from build123d import *

# Parameters (mm, degrees)
F2_SIZE  = 1
F3_R     = 0.99999
F4_R     = 2
F5_R     = 2
F6_DEPTH = 30.0010001


# Not quite as in the source:
# - a fillet or chamfer is up to 0.001 mm smaller than in the source, because OpenCascade refuses the exact size


with BuildPart() as f1:
    # F0 (on Front) → F1 (revolve)
    with BuildSketch(Plane.XZ):
        Polygon((0, 30), (0, 20), (1, 20), (1, 10), (12, 10), (12, 17.5), (6.3493649054, 17.5), (3, 30), align=None)
    revolve(axis=Axis((7.1844396027, 0, 0), (1, 0, 0)))

    # F2
    f2_edges = [f1.edges().sort_by_distance(p)[0] for p in [
        (12, 0, -17.5),
    ]]
    chamfer(f2_edges, length=F2_SIZE)

    # F3 (radius 1 in the source; OpenCascade refuses exactly that, so slightly less here)
    f3_edges = [f1.edges().sort_by_distance(p)[0] for p in [
        (3, 0, -30),
        (1, 0, -20),
    ]]
    fillet(f3_edges, radius=F3_R)

    # F4
    f4_edges = [f1.edges().sort_by_distance(p)[0] for p in [
        (6.349365, 0, -17.5),
    ]]
    fillet(f4_edges, radius=F4_R)

    # F5 (on Top) → F6 (cut, through all)
    with BuildSketch(Plane.XY):
        with Locations((8, 0)):
            Circle(F5_R)
    extrude(amount=F6_DEPTH, mode=Mode.SUBTRACT)


solid = f1.part
Geometry check sheet. Reference: the model listing, model coordinates, mm. A direction names the side the tool comes from. Coordinates: 2 decimals unless noted, no trailing zeros. Order: outer loops, then holes, each group sorted by start corner. A loop starts at its lowest first (then second) coordinate and runs counter-clockwise, first axis right, second up. Notation, with made-up numbers: M -8.5,24 L 14.5,24 A17 cw 14.5,51 Z; hole C 12.25,-14.5 d5. An arc over 180 degrees is marked long. Use CSV: the item, a comma, the result in double quotes.
Item 1: Gauge pin test, flat ends, axial feed: pin 1 Ø6 at (x, y) = (10.5, 11) entering from +Z; pin 2 Ø4 at (x, y) = (8.5, -8) entering from +Z; pin 3 Ø5 at (x, z) = (3.5, 2.5) entering from +Y. Record the tip position at first contact, or that the pin passes through.
Returned:
pin 1,"stops at z = 15.56"
pin 2,"stops at z = 16.44"
pin 3,"stops at y = 30"
Item 2: Tool access check on faces 1 (the cylindrical face through (9.42, 10.648, -13.887)), 2 (the cylindrical face through (1.101, 11.49, 27.712)), 3 (the flat face through (1, 8, 8)). Record the directions out of +Z, -Z, +X, -X, +Y, -Y that give a thin tool (end or side, any length) a straight path to the whole face; none if there is none.
Returned:
face 1,"+X"
face 2,"+X, -X"
face 3,"-X"
Item 3: Mould release check, pull along X, two halves, no side actions. Record for faces 4 (the cylindrical face through (6, 0, 14)), 5 (the flat face through (12, 11, 0)), 6 (the flat face through (0, 20, 6)): pulls with the +X half, pulls with the -X half, needs draft (parallel to the pull), parting line crosses it, or undercut.
Returned:
face 4,"undercut"
face 5,"pulls with the +X half"
face 6,"pulls with the -X half"
Item 4: Cross-section at C-C on x = 9.25. Record the cut outline in (y, z), then the cut area to 3 significant figures.
Returned:
outline,"M -1.56,9.88 L -1.56,17.43 A17.5 ccw long 1.56,17.43 L 1.56,9.88 A10 cw long Z"
area,"624 mm2"
Item 5: Cross-section at A-A on y = 0. Give the number of separate pieces and of enclosed holes in the cut face, then the cut area to 3 significant figures.
Returned:
separate pieces,"3"
enclosed holes,"0"
area,"246 mm2"
Item 6: Cross-section at B-B on x = 4.5. Record the cut outline in (y, z), then the cut area to 3 significant figures.
Returned:
outline,"C 0,0 d48.8; hole C 0,0 d20"
area,"1,560 mm2"
Item 7: Thickness scan on line 1 along X through (y, z) = (0, 12.5); line 2 along X through (y, z) = (17, -8); line 3 along X through (y, z) = (-8, -8.5). Record the ranges inside material, lowest first.
Returned:
line 1,"x = 1 to 6, 10 to 12"
line 2,"x = 1 to 6.01"
line 3,"x = 1 to 12"
